```python
from build123d import *

# Parameters (mm, degrees)
SKETCH1_W           = 245
SKETCH1_H           = 15
SKETCH1_R           = 3.25
BOSS_EXTRUDE1_DEPTH = 2
SKETCH2_W           = 5
SKETCH2_H           = 5
CUT_EXTRUDE1_DEPTH  = 10


with BuildPart() as part:
    # Sketch1 → Boss-Extrude1 (new body)
    with BuildSketch(Plane.XY):
        Rectangle(SKETCH1_W, SKETCH1_H)
        with Locations((-112.5, 0)):
            Circle(SKETCH1_R, mode=Mode.SUBTRACT)
        with Locations((112.5, 0)):
            Circle(SKETCH1_R, mode=Mode.SUBTRACT)
    extrude(amount=BOSS_EXTRUDE1_DEPTH)

    # Sketch2 → Cut-Extrude1 (cut)
    with BuildSketch(Plane.XY.offset(2)):
        with Locations((-40, -2.5)):
            Rectangle(SKETCH2_W, SKETCH2_H)
        with Locations((40, -2.5)):
            Rectangle(SKETCH2_W, SKETCH2_H)
    extrude(amount=-CUT_EXTRUDE1_DEPTH, mode=Mode.SUBTRACT)


solid = part.part
```
Geometry check sheet. Reference: the model listing, model coordinates, mm. Give positions to 0.01 mm unless a question says otherwise; leave off trailing zeros. Order: outer loops, then holes, each group sorted by start corner. A loop starts at its lowest first (then second) coordinate and runs counter-clockwise, first axis right, second up. Notation, with made-up numbers: (80, 36.25) -> (84, 36.25) arc R18 cw to (84, 48.25) -> close; hole circle Ø1 at (-21.75, 3). An arc over 180 degrees is marked (long way). Write each question's results on one line, items separated by ' | '. Start each with the question number.
(1) Sectioned sample at B-B (x = -112.5). Enter the section's corners in (y, z), plus the area to 3 significant figures.
(2) Scan lines: line 1 (X direction, y = 0.5, z = 1.2); line 2 (X direction, y = -4.25, z = 0.85); line 3 (Y direction, x = -112.5, z = 1.4). Record each from-to range of solid material in increasing order.
(3) Gauge pin test, flat end, axial feed: P1, Ø3, axis at x = -40, y = -5, coming from the -Z side. Record the tip position at first contact, or that the pin passes through.
(4) Mould release check, pull along X, two halves, no side actions. Record for faces 1 (the face through (-2, 0, 0)), 2 (the face through (-115.747, 0.143, 0.986)), 3 (the face through (109.253, 0.143, 0.986)): pulls with the +X half, pulls with the -X half, needs draft (parallel to the pull), parting line crosses it, or undercut.
(5) Sectioned sample at A-A (z = 0.3). Enter the section's corners in (x, y).
Answer below:
1) outline: (-7.5, 0) -> (-3.25, 0) -> (-3.25, 2) -> (-7.5, 2) -> close; (3.25, 0) -> (7.5, 0) -> (7.5, 2) -> (3.25, 2) -> close | area: 17.0 mm2
2) line 1: -122.5 to -115.71, -109.29 to 109.29, 115.71 to 122.5 | line 2: -122.5 to -42.5, -37.5 to 37.5, 42.5 to 122.5 | line 3: -7.5 to -3.25, 3.25 to 7.5
3) P1: z = 0
4) face 1: needs draft | face 2: undercut | face 3: undercut
5) outline: (-122.5, -7.5) -> (122.5, -7.5) -> (122.5, 7.5) -> (-122.5, 7.5) -> close; hole circle Ø6.5 at (-112.5, 0); hole (-42.5, -5) -> (-37.5, -5) -> (-37.5, 0) -> (-42.5, 0) -> close; hole (37.5, -5) -> (42.5, -5) -> (42.5, 0) -> (37.5, 0) -> close; hole circle Ø6.5 at (112.5, 0)
